```python
from build123d import *

# Parameters (mm, degrees)
SKETCH1_R                  = 2.0025
BOSS_EXTRUDE1_DEPTH        = 7.5
M3X0_5_TAPPED_HOLE1_REACH  = 10.922
M3X0_5_TAPPED_HOLE1_BORE_R = 1.2525
FILLET1_R                  = 0.25


with BuildPart() as part:
    # Sketch1 → Boss-Extrude1 (new body)
    with BuildSketch(Plane(origin=(0, 0, 0), x_dir=(1, 0, 0), z_dir=(0, 1, 0))):
        Polygon((0, 4), (-3.464101615, 2), (-3.464101615, -2), (0, -4), (3.464101615, -2), (3.464101615, 2), align=None)
        with Locations(Location((0, 0, 0), (0, 0, 270))):
            Circle(SKETCH1_R, mode=Mode.SUBTRACT)
    extrude(amount=BOSS_EXTRUDE1_DEPTH)

    # M3x0.5 Tapped Hole1 bore (on position points) → M3x0.5 Tapped Hole1 (cut, up to next)
    with BuildSketch(Plane(origin=(3.464101615, 3.55, 0), x_dir=(0, 0, 1), z_dir=(1, 0, 0)), mode=Mode.PRIVATE) as m3x0_5_tapped_hole1_sk1:
        Circle(M3X0_5_TAPPED_HOLE1_BORE_R)
    m3x0_5_tapped_hole1_tool1 = extrude(m3x0_5_tapped_hole1_sk1.sketch, amount=-M3X0_5_TAPPED_HOLE1_REACH, mode=Mode.PRIVATE) & part.part
    add(m3x0_5_tapped_hole1_tool1.solids().sort_by_distance((3.464102, 3.55, 0))[0], mode=Mode.SUBTRACT)

    # Fillet1
    fillet1_edges = [part.edges().sort_by_distance(p)[0] for p in [
        (-3.464101615, 7.5, 0),
        (-1.732050808, 7.5, 3),
        (1.732050808, 7.5, 3),
        (3.464101615, 7.5, 0),
        (1.732050808, 7.5, -3),
        (3.464101615, 0, 0),
        (1.732050808, 0, 3),
        (-1.732050808, 0, 3),
        (-1.732050808, 7.5, -3),
        (-3.464101615, 0, 0),
        (-1.732050808, 0, -3),
        (1.732050808, 0, -3),
    ]]
    fillet(fillet1_edges, radius=FILLET1_R)


solid = part.part
```
Design review of the part built by this model. Coordinates are the model's own, in mm. Give positions to 0.01 mm unless a question says otherwise; leave off trailing zeros. Order: outer loops, then holes, each group sorted by start corner. A loop starts at its lowest first (then second) coordinate and runs counter-clockwise, first axis right, second up. Notation, with made-up numbers: (86, 57) -> (117, 57) arc R33 ccw to (117, 96) -> close; hole circle Ø7 at (-31.75, 74). An arc over 180 degrees is marked (long way). Write item = value, one per line. Start each with the question number.
(1) For pin 1 (3 mm diameter, centred on x = 1, y = 4.5, fed in from +Z), flat-tipped, find the tip position at first contact; note if it passes through.
(2) We need section A-A on z = 0. Write out the cut boundary in (x, y).
(3) We need section D-D on y = 4.5. Write out the cut boundary in (x, z) (1 decimal), plus the area to 3 significant figures.
(4) We need section B-B on y = 6.5. Write out the cut boundary in (x, z) (1 decimal), plus the area to 3 significant figures.
(5) Mouldability with a two-part tool opening along Y and no side actions: class faces 1 (the face through (1, 7.5, 2)), 2 (the face through (2.53, 2.49, 0.67)), 3 (the face through (-1.708, 3.701, -3.014)) as +Y half, -Y half, draft (parallel to the pull), parting line (faces both ways), or undercut.
(6) We need section C-C on y = 3.55. Write out the cut boundary in (x, z) (1 decimal).
(7) To check wall thickness, follow line 1 along Y through (x, z) = (2.75, 0); line 2 along X through (y, z) = (5.5, 0); line 3 along Z through (x, y) = (1, 6.75). State the ranges of each line that lie inside material, in increasing order.
Numbers:
q1.pin_1 = 4
q2.outline = (-3.46, 0.25) arc R0.25 ccw to (-3.21, 0) -> (-2, 0) -> (-2, 7.5) -> (-3.21, 7.5) arc R0.25 ccw to (-3.46, 7.25) -> close; (2, 0) -> (3.21, 0) arc R0.25 ccw to (3.46, 0.25) -> (3.46, 2.3) -> (2, 2.3) -> close; (2, 4.8) -> (3.46, 4.8) -> (3.46, 7.25) arc R0.25 ccw to (3.21, 7.5) -> (2, 7.5) -> close
q3.outline = (-3.5, -2) -> (0, -4) -> (3.5, -2) -> (3.5, -0.8) -> (1.8, -0.8) arc R2 cw (long way) to (1.8, 0.8) -> (3.5, 0.8) -> (3.5, 2) -> (0, 4) -> (-3.5, 2) -> close
q3.area = 26.5 mm^2
q4.outline = (-3.5, -2) -> (0, -4) -> (3.5, -2) -> (3.5, 2) -> (0, 4) -> (-3.5, 2) -> close; hole circle Ø4 at (0, 0)
q4.area = 29.0 mm^2
q5.face_1 = +Y half
q5.face_2 = undercut
q5.face_3 = draft
q6.outline = (-3.5, -2) -> (0, -4) -> (3.5, -2) -> (3.5, -1.3) -> (1.6, -1.3) arc R2 cw (long way) to (1.6, 1.3) -> (3.5, 1.3) -> (3.5, 2) -> (0, 4) -> (-3.5, 2) -> close
q7.line_1 = 0 to 2.3, 4.8 to 7.5
q7.line_2 = -3.46 to -2, 2 to 3.46
q7.line_3 = -3.42 to -1.73, 1.73 to 3.42
